Here's how the part is built. I have some questions about the finished solid (model axes, mm). A direction names the side the tool comes from. Round coordinates to 2 decimals unless told otherwise and drop trailing zeros. Write each loop counter-clockwise with the first axis right and the second up, starting at its lowest first coordinate (ties: lowest second). Pieces come first, ordered by that corner, then holes. Notation, with made-up numbers: (48, -4) - (73, -4) arc R20 ccw to (73, 31) - close; hole circle Ø8 at (43, -3.75). An arc over 180 degrees is marked (long way). One line per item, written item: value. Start each with the question number.
Item 1: Imagine slicing it at D-D, the plane x = 2.5. Please give me the cut outline in (y, z), then the cut area to 3 significant figures.
Item 2: For P1, Ø1.5, axis at y = -5.5, z = 3.5, coming from the -X side; P2, Ø1.7, axis at y = -8.5, z = 6, coming from the +X side; P3, Ø3, axis at x = -16, y = 1.5, coming from the +Z side; P4, Ø6, axis at x = 12, y = -3.5, coming from the +Z side, each with a flat end and sliding along its axis, tell me the tip position at first contact or that it passes through.
Item 3: Thinking about a two-plate mould opening in X: for faces 1 (the face through (-17, 1, 5.08)), 2 (the face through (-1, -7.62, 4)), 3 (the face through (-3.74, -3.72, 11.4)), which applies, released by +X, released by -X, zero draft, split by the parting line, or undercut?
Item 4: Imagine slicing it at C-C, the plane y = 1.25. Please give me the cut outline in (x, z).
Item 5: Imagine slicing it at B-B, the plane x = 13.5. Please give me the cut outline in (y, z).
Item 6: Imagine slicing it at A-A, the plane y = -7. Please give me the cut outline in (x, z).
Item 7: If I drill on line 1 (Z direction, x = 0, y = -8.5); line 2 (Y direction, x = 10.5, z = 1.75); line 3 (Z direction, x = 11, y = -8.75), over which ranges is the centre line in solid material (lowest first)?
Item 8: For faces 4 (the face through (28.401, -4, 2)), 5 (the face through (-0.07, -8.91, 4.89)), 6 (the face through (-5.866, 1, 6)), 7 (the face through (-1, 1, 0)), 8 (the face through (16, -9, 5.08)), which set-ups out of +Z, -Z, +X, -X, +Y, -Y let a thin tool reach every point of the face, with its end or its side?
```python
from build123d import *

# Parameters (mm, degrees)
F0_W        = 22.3517898379
F0_H        = 5.08
F0_W_2      = 24.1537776476
F0_W_3      = 6.0488656163
F0_H_2      = 4.7264951599
F0_W_4      = 5.8655668981
F1_DEPTH    = 7.62
F2_T        = 2.54
F3_R        = 0.5
F4_DEPTH    = 8.10174
F6_T1_DEPTH = 38.1
F6_T3_DEPTH = 38.1
F6_T5_DEPTH = 38.1
F6_T7_DEPTH = 38.1
F7_DEPTH    = 7.36236


# Not quite as in the source:
# - a fillet or chamfer that OpenCascade refuses, or shapes differently, is made with other operations: its cross-section is extruded or revolved along the edge and cut away or added
# - a feature of the source that left no trace in its solid (it failed there, or was rolled back) is left out


with BuildPart() as f1:
    # F0 (on Front) → F1 (new body)
    with BuildSketch(Plane.XZ):
        Polygon((-5.8655668981, 0), (0, 0), (6.0488656163, 0), (6.0488656163, 5.08), (0, 5.08), (-5.8655668981, 5.08), align=None)
        with Locations((17.2247605353, 2.54)):
            Rectangle(F0_W, F0_H)
        with Locations((-17.942455722, 2.54)):
            Rectangle(F0_W_2, F0_H)
        with Locations((3.0244328082, 7.4432475799)):
            Rectangle(F0_W_3, F0_H_2)
        with Locations((-2.9327834491, 7.4432475799)):
            Rectangle(F0_W_4, F0_H_2)
    extrude(amount=F1_DEPTH)

    # F2
    f2_openings = [f1.faces().sort_by_distance(p)[0] for p in [
        (-17.942456, -3.81, 5.08),
        (-0.809345, -3.81, 0),
        (17.224761, -3.81, 5.08),
        (6.048866, -3.81, 7.443248),
        (-5.865567, -3.81, 7.443248),
    ]]
    offset(amount=F2_T, openings=f2_openings, kind=Kind.INTERSECTION)

    # F3 (on face) → F4 (cut)
    with BuildSketch(Plane.XZ.offset(10.16)):
        with Locations((0, 4.3936586007)):
            Circle(F3_R)
    extrude(amount=-F4_DEPTH, mode=Mode.SUBTRACT)

    # F6: fillet of radius 5.08 on 6 edges, made by hand

    # F6_s2 → F6_t1 (cut)
    with BuildSketch(Plane.XZ.offset(-15.24)):
        with BuildLine():
            ThreePointArc((25.8606554542, 5.08), (29.4527579027, 3.5921024484), (30.9406554542, 0))
            Line((30.9406554542, 0), (31.0422554542, 0))
            Line((31.0422554542, 0), (31.0422554542, 5.1816))
            Line((31.0422554542, 5.1816), (25.8606554542, 5.1816))
            Line((25.8606554542, 5.1816), (25.8606554542, 5.08))
        make_face()
    extrude(amount=F6_T1_DEPTH, mode=Mode.SUBTRACT)

    # F6_s4 → F6_t3 (cut)
    with BuildSketch(Plane.XZ.offset(-15.24)):
        with BuildLine():
            ThreePointArc((-27.4793445458, 5.08), (-31.0714469942, 3.5921024484), (-32.5593445458, 0))
            Line((-32.5593445458, 0), (-32.6609445458, 0))
            Line((-32.6609445458, 0), (-32.6609445458, 5.1816))
            Line((-32.6609445458, 5.1816), (-27.4793445458, 5.1816))
            Line((-27.4793445458, 5.1816), (-27.4793445458, 5.08))
        make_face()
    extrude(amount=F6_T3_DEPTH, mode=Mode.SUBTRACT)

    # F6_s6 → F6_t5 (cut)
    with BuildSketch(Plane.XZ.offset(-15.24)):
        with BuildLine():
            ThreePointArc((6.0488656163, 7.2664951599), (4.5609680647, 10.8585976083), (0.9688656163, 12.3464951599))
            Line((0.9688656163, 12.3464951599), (0.9688656163, 12.4480951599))
            Line((0.9688656163, 12.4480951599), (6.1504656163, 12.4480951599))
            Line((6.1504656163, 12.4480951599), (6.1504656163, 7.2664951599))
            Line((6.1504656163, 7.2664951599), (6.0488656163, 7.2664951599))
        make_face()
    extrude(amount=F6_T5_DEPTH, mode=Mode.SUBTRACT)

    # F6_s8 → F6_t7 (cut)
    with BuildSketch(Plane.XZ.offset(-15.24)):
        with BuildLine():
            ThreePointArc((-5.8655668981, 7.2664951599), (-4.3776693466, 10.8585976083), (-0.7855668981, 12.3464951599))
            Line((-0.7855668981, 12.3464951599), (-0.7855668981, 12.4480951599))
            Line((-0.7855668981, 12.4480951599), (-5.9671668981, 12.4480951599))
            Line((-5.9671668981, 12.4480951599), (-5.9671668981, 7.2664951599))
            Line((-5.9671668981, 7.2664951599), (-5.8655668981, 7.2664951599))
        make_face()
    extrude(amount=F6_T7_DEPTH, mode=Mode.SUBTRACT)

    # F3 (on face) → F7 (cut)
    with BuildSketch(Plane.XZ.offset(10.16)):
        with Locations((0, 4.3936586007)):
            Circle(F3_R)
    extrude(amount=-F7_DEPTH, mode=Mode.SUBTRACT)


solid = f1.part
```
Values follow:
1. outline: (-10.16, 0) - (-7.62, 0) - (-7.62, 9.81) - (0, 9.81) - (0, 0) - (2.54, 0) - (2.54, 12.11) - (-10.16, 12.11) - close
1. area: 79.1 mm^2
2. P1: stops at x = -31.75
2. P2: stops at x = 6.05
2. P3: stops at z = 5.08
2. P4: passes through
3. face 1: zero draft
3. face 2: undercut
3. face 3: released by -X
4. outline: (-32.56, 0) - (30.94, 0) arc R5.08 ccw to (25.86, 5.08) - (6.05, 5.08) - (6.05, 7.27) arc R5.08 ccw to (0.97, 12.35) - (-0.79, 12.35) arc R5.08 ccw to (-5.87, 7.27) - (-5.87, 5.08) - (-27.48, 5.08) arc R5.08 ccw to start
5. outline: (-10.16, 0) - (-7.62, 0) - (-7.62, 5.08) - (-10.16, 5.08) - close; (0, 0) - (2.54, 0) - (2.54, 5.08) - (0, 5.08) - close
6. outline: (-32.56, 0) - (-30.02, 0) - (-30.02, 4.4) arc R5.08 ccw to start; (-5.18, 9.81) - (5.37, 9.81) arc R5.08 ccw to (0.97, 12.35) - (-0.79, 12.35) arc R5.08 ccw to start; (28.4, 0) - (30.94, 0) arc R5.08 ccw to (28.4, 4.4) - close
7. line 1: z = 0 to 3.89, 4.89 to 12.35
7. line 2: y = -10.16 to -7.62, 0 to 2.54
7. line 3: z = 0 to 5.08
8. face 4: +Z, -Z
8. face 5: -Y
8. face 6: +Z, -X, +Y, -Y
8. face 7: -Z, +X, -X, +Y, -Y
8. face 8: +Z, +X, +Y, -Y
